Autodesk Inventor part; units mm, degrees
ref_plane "YZ Plane" through (0, 0, 0) normal (1, 0, 0) x (0, 1, 0)
ref_plane "XZ Plane" through (0, 0, 0) normal (0, 1, 0) x (-1, 0, 0)
ref_plane "XY Plane" through (0, 0, 0) normal (0, 0, 1) x (1, 0, 0)
sketch "Esquisse5" plane through (0, 0, 0) normal (1, 0, 0) x (0, 1, 0)
  line L0 (0, 0) -> (28, 0)
  line L1 (28, 0) -> (28, -17)
  line L2 (28, -17) -> (0, -17)
  line L3 (0, -17) -> (0, 0)
  line L4 (0, 0) -> (0, -2)
  line L5 (0, -2) -> (2, -2)
  line L6 (28, -17) -> (28, -15)
  line L7 (28, -15) -> (26, -15)
  line L8 (26, -15) -> (2, -15)
  line L9 (2, -15) -> (2, -2)
  line L10 (2, -2) -> (26, -2)
  line L11 (26, -2) -> (26, -15)
  dimension "d20" = 28
  dimension "d21" = 17
  dimension "d22" = 2
  dimension "d23" = 2
  dimension "d24" = 2
  dimension "d25" = 2
extrude "Extrusion4" add sketch "Esquisse5" along normal blind 23.4 contours L0 L1 L7 L11 L10 L5 L3 | L5 L9 L8 L7 L1 L2 L3
sketch "Esquisse6" plane through (0, 0, 0) normal (-1, 0, 0) x (0, 0, 1)
  line L0 (-15, 2) -> (-2, 2)
  line L1 (-2, 2) -> (-2, 26)
  line L2 (-15, 2) -> (-2, 2)
  line L3 (-2, 2) -> (-2, 26)
  line L4 (-2, 26) -> (-15, 26)
  line L5 (-15, 26) -> (-15, 2)
  point P0 (0, 0)
extrude "Extrusion5" add sketch "Esquisse6" against normal blind 2
sketch "Esquisse7" plane through (2, 0, 0) normal (1, 0, 0) x (0, 0, -1)
  line L0 (15, 2) -> (2, 2)
  line L1 (2, 2) -> (2, 19.4)
  line L2 (2, 2) -> (2, 26)
  line L3 (2, 19.4) -> (2, 21.5)
  line L4 (2, 21.5) -> (2, 26)
  line L5 (2, 21.5) -> (2, 26)
  line L6 (15, 2) -> (2, 2)
  line L7 (2, 2) -> (2, 19.4)
  line L8 (2, 19.4) -> (15, 19.4)
  line L9 (15, 19.4) -> (15, 2)
  line L10 (2, 26) -> (15, 26)
  line L11 (15, 26) -> (2, 26)
  line L12 (2, 26) -> (2, 21.5)
  line L13 (2, 21.5) -> (15, 21.5)
  line L14 (15, 21.5) -> (15, 26)
  point P0 (0, 0)
  dimension "d30" = 17.4
  dimension "d31" = 2.1
extrude "Extrusion6" add sketch "Esquisse7" along normal blind 4.5
sketch "Esquisse8" plane through (6.5, 0, 0) normal (1, 0, 0) x (0, 0, -1)
  line L0 (15, 26) -> (15, 2)
  line L1 (2, 2) -> (15, 2)
  line L2 (15, 2) -> (15, 10)
  line L3 (15, 10) -> (2, 10)
  line L4 (2, 10) -> (2, 2)
  point P0 (0, 0)
  dimension "d34" = 8
extrude "Extrusion7" cut sketch "Esquisse8" against normal up to next
sketch "Esquisse9" plane through (0, 28, 0) normal (0, 1, 0) x (1, 0, 0)
  line L0 (22.4357, 15) -> (23.4, 15)
  line L1 (22.4357, 2) -> (23.4, 2)
  arc A0 (23.4, 15) -> (23.4, 2) centre (22.9179, 8.5) ccw
  line L2 (23.4, 2) -> (23.4, 15)
  line L3 (23.4, 15) -> (23.4, 2)
  line L4 (23.4, 2) -> (23.4, 15)
  line L5 (23.4, 0) -> (23.4, 2)
  point P0 (0, 0)
extrude "Extrusion8" cut sketch "Esquisse9" against normal blind 4.5 contours L0 L2 L1 A0
sketch "Esquisse10" plane through (6.5, 26, -15) normal (0, -1, 0) x (1, 0, 0)
  line L0 (0, 13) -> (0, 0)
  line L1 (0, 6.5) -> (7, 6.5)
  line L2 (7, 6.5) -> (10.25, 6.5)
  circle A0 centre (10.25, 6.5) radius 3.25
  point P0 (-6.5, 15)
  dimension "d39" = 7
  dimension "d41" = 6.5
extrude "Extrusion9" cut sketch "Esquisse10" against normal up to next
sketch "Esquisse11" plane through (0, 0, 0) normal (-1, 0, 0) x (0, 0, 1)
  line L0 (-17, 28) -> (-15, 28)
  line L1 (0, 0) -> (-17, 0)
  line L2 (-17, 0) -> (-17, 28)
  line L3 (-17, 28) -> (0, 28)
  line L4 (0, 28) -> (0, 0)
  line L5 (-2, 2) -> (-2, 28)
  line L6 (-15, 26) -> (-15, 21.5)
  line L7 (-2, 2) -> (-15, 2)
  line L8 (-15, 2) -> (-15, 26)
  line L9 (-15, 26) -> (-2, 26)
  line L10 (-2, 26) -> (-2, 2)
extrude "Extrusion10" add sketch "Esquisse11" along normal blind 13.5
sketch "Esquisse12" plane through (-13.5, 0, 0) normal (-1, 0, 0) x (0, 0, 1)
  line L0 (0, 0) -> (-17, 0)
  line L1 (-17, 0) -> (-17, -10)
  line L2 (-17, -10) -> (0, -10)
  line L3 (0, -10) -> (0, 0)
  line L4 (0, 28) -> (0, 0)
  line L5 (0, 28) -> (-17, 28)
  line L6 (-17, 28) -> (-17, 38)
  line L7 (-17, 38) -> (0, 38)
  line L8 (0, 38) -> (0, 28)
  dimension "d46" = 17
  dimension "d47" = 10
  dimension "d50" = 17
  dimension "d51" = 10
extrude "Extrusion11" add sketch "Esquisse12" against normal blind 3
fillet "Congé1" radius 5 1 edges at (-12, 38, -17)
fillet "Congé2" radius 5 3 edges at (-12, 38, 0) (-12, -10, -17) (-12, -10, 0)
sketch "Esquisse13" plane through (-10.5, 0, 0) normal (1, 0, 0) x (0, 0, -1)
  line L0 (5, -10) -> (12, -10)
  line L1 (8.5, -10) -> (8.5, -5)
  line L2 (8.5, -5) -> (8.5, 33)
  circle A0 centre (8.5, -5) radius 2
  circle A1 centre (8.5, 33) radius 2
  point P0 (0, 0)
  dimension "d54" = 5
  dimension "d55" = 38
  dimension "d56" = 4
  dimension "d57" = 4
extrude "Extrusion12" cut sketch "Esquisse13" against normal up to next
fillet "Congé3" radius 1 14 edges at (6.45, 28, -17) (6.45, 0, -17) (6.45, 0, 0) (6.45, 28, 0) (-10.5, 36.5355, -15.5355) (-10.5, 38, -8.5) (-10.5, 36.5355, -1.4645) (-10.5, 30.5, 0) (-10.5, 30.5, -17) (-10.5, -8.5355, -15.5355) (-10.5, -10, -8.5) (-10.5, -8.5355, -1.4645) (-10.5, -2.5, 0) (-10.5, -2.5, -17)
properties part number "Support bas servomoteur"
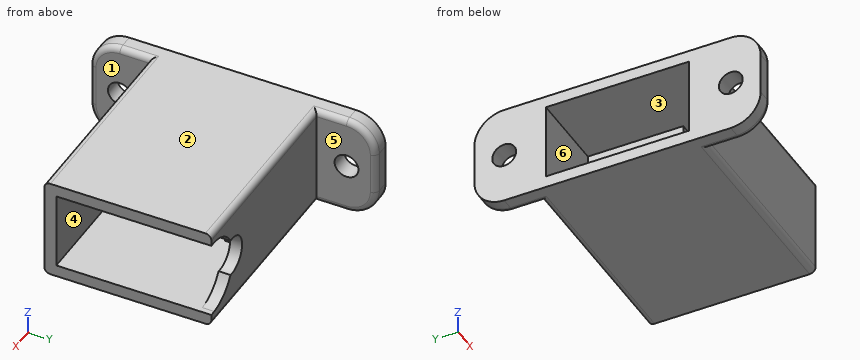
Verification items for the finished model (mm, model axes). Face numbers are marked on the shaded views. A direction names the side the tool comes from. Round coordinates to 2 decimals unless told otherwise and drop trailing zeros. Loops run counter-clockwise (first coordinate to the right, second up) from the corner with the lowest first, then second, coordinate; pieces in that order, holes last. Notation, with made-up numbers: (50, 72.25) - (100, 72.25) arc R15 ccw to (100, 83.25) - close; hole circle Ø4 at (69, -12). An arc over 180 degrees is marked (long way). Write item = value, one per line.
Q1. Sectioned sample at C-C on y = 3.5. Record the boundary of the cut face in (x, z), plus the area to 3 significant figures.
Here are the results:
outline = (-13.5, -17) - (23.4, -17) - (23.4, -15) - (-13.5, -15) - close; (-13.5, -2) - (23.4, -2) - (23.4, 0) - (-13.5, 0) - close
area = 148 mm^2
Q2. Sectioned sample at A-A on x = 8. Record the boundary of the cut face in (y, z).
Here are the results:
outline = (0, -16) arc R1 ccw to (1, -17) - (27, -17) arc R1 ccw to (28, -16) - (28, -1) arc R1 ccw to (27, 0) - (1, 0) arc R1 ccw to (0, -1) - close; hole (2, -15) - (26, -15) - (26, -2) - (2, -2) - close
Q3. Tool access check on the marked faces 4, 5 and 6. Record the directions out of +Z, -Z, +X, -X, +Y, -Y that give a thin tool (end or side, any length) a straight path to the whole face; none if there is none.
Here are the results:
face_4 = +X, -X
face_5 = +Z, -Z, +X, +Y
face_6 = -X
Q4. Sectioned sample at B-B on z = -8.5. State how many separate pieces and enclosed holes the cut face has, plus the area to 3 significant figures.
Here are the results:
separate_pieces = 4
enclosed_holes = 0
area = 258 mm^2
Q5. Material ranges on L1, parallel to Y at x = -12.1, z = -8.5; L2, parallel to Z at x = 21.5, y = 25; L3, parallel to Y at x = -1, z = -5.25, recorded low to high.
Here are the results:
L1 = -10 to -7, -3 to 2, 26 to 31, 35 to 38
L2 = -17 to -15, -2 to 0
L3 = 0 to 2, 26 to 28
Q6. Mould release check, pull along Z, two halves, no side actions. Record for the marked faces 1, 2 and 3: +Z half, -Z half, draft (parallel to the pull), parting line (faces both ways), or undercut.
Here are the results:
face_1 = draft
face_2 = +Z half
face_3 = undercut
Q7. Sectioned sample at D-D on y = -2. Record the boundary of the cut face in (x, z).
Here are the results:
outline = (-13.5, -17) - (-11.5, -17) arc R1 ccw to (-10.5, -16) - (-10.5, -1) arc R1 ccw to (-11.5, 0) - (-13.5, 0) - close
Q8. Depth check by flat-ended pin: pin 1 (6.5 mm diameter, centred on x = -4, z = -10, fed in from -Y); pin 2 (2.5 mm diameter, centred on y = 34, z = -9, fed in from +X); pin 3 (2 mm diameter, centred on x = -1, z = -8.5, fed in from +Y); pin 4 (1.5 mm diameter, centred on y = 8.5, z = -5.5, fed in from -X). Enter the tip coordinate at first touch or a pass-through.
Here are the results:
pin_1 = 0
pin_2 = -10.5
pin_3 = 28
pin_4 = through
